Here's how the part is built. I have some questions about the finished solid (model axes, mm). A direction names the side the tool comes from. Coordinates: 2 decimals unless noted, no trailing zeros. Loops run counter-clockwise (first coordinate to the right, second up) from the corner with the lowest first, then second, coordinate; pieces in that order, holes last. Notation, with made-up numbers: (49.25, 85.5) -> (71.25, 85.5) arc R21 cw to (71.25, 101.5) -> close; hole circle Ø8 at (22.25, 38.5). An arc over 180 degrees is marked (long way). Use CSV: the item, a comma, the result in double quotes. Start each with the question number.
Autodesk Inventor part; units mm, degrees
ref_plane "YZ Plane" through (0, 0, 0) normal (1, 0, 0) x (0, 1, 0)
ref_plane "XZ Plane" through (0, 0, 0) normal (0, 1, 0) x (-1, 0, 0)
ref_plane "XY Plane" through (0, 0, 0) normal (0, 0, 1) x (1, 0, 0)
sketch "Sketch5" plane through (0, 0, 0) normal (0, 0, 1) x (1, 0, 0)
  line L0 (52.8, -15.6) -> (52.8, -10.6)
  line L1 (52.8, -10.6) -> (49.8, -10.6)
  line L2 (49.8, -10.6) -> (49.8, -12.55)
  line L3 (44, -12.55) -> (44, -3.05)
  line L4 (49.8, -3.05) -> (49.8, -5)
  line L5 (49.8, -5) -> (52.8, -5)
  line L6 (52.8, -5) -> (52.8, 0)
  line L7 (52.8, 0) -> (7.8, 0)
  line L8 (44, -3.05) -> (49.8, -3.05)
  line L9 (44, -12.55) -> (49.8, -12.55)
  line L10 (52.8, -15.6) -> (7.8, -15.6)
  arc A0 (7.8, 0) -> (7.8, -15.6) centre (7.8, -7.8) ccw
  point P0 (0, 0)
  dimension "d41" = 5.8
  dimension "d48" = 44
  dimension "d50" = 3
  dimension "d63" = 45
  dimension "d67" = 15.6
  dimension "d71" = 0
  dimension "d72" = 36.2
  dimension "d87" = 5.6
  dimension "d88" = 9.5
extrude "Extrusion2" add sketch "Sketch5" along normal blind 12
sketch "Sketch11" plane through (0, 0, 12) normal (0, 0, 1) x (1, 0, 0)
  line L0 (52.8, 0) -> (7.8, 0)
  line L1 (13.859, 0) -> (15.2481, -7.8785)
  line L2 (15.2481, -7.8785) -> (0.476, -10.4832)
  arc A0 (7.8, 0) -> (7.8, -15.6) centre (7.8, -7.8) ccw
  point P0 (0, 0)
  dimension "d95" = 100
  dimension "d96" = 8
  dimension "d97" = 15
extrude "Extrusion7" cut sketch "Sketch11" along normal blind 10 from surface at -12
sketch "Sketch14" plane through (0, 0, 12) normal (0, 0, 1) x (1, 0, 0)
  line L0 (2.8531, 4.8295) -> (7.1439, -19.5045)
  line L1 (7.1439, -19.5045) -> (-13.8708, -23.21)
  line L2 (-13.8708, -23.21) -> (-18.1616, 1.124)
  line L3 (-18.1616, 1.124) -> (2.8531, 4.8295)
  line L4 (13.859, 0) -> (15.2481, -7.8785)
  point P0 (0, 0)
  dimension "d111" = 10
extrude "Extrusion10" cut sketch "Sketch14" against normal through all
fillet "Fillet2" radius 15 1 edges at (6.4341, -15.4795, 6)
equation "\"l1\" = 8"
properties part number "Finray_test_8_Kerbe_10deg_V4"
1) Which directions (+Z, -Z, +X, -X, +Y, -Y) give clear straight access to the entire face, cutting with the end or side of a thin tool? Please do faces 4 (the face through (4.077, -2.113, 11.014)), 5 (the face through (44, -8, 6)), 6 (the face through (14.544, -3.884, 4.93)), 7 (the face through (51, -5, 6)), 8 (the face through (52.8, -3, 6)).
2) I want a section at A-A, the plane y = -4. Please give me the cut outline in (x, z).
3) For P1, Ø3, axis at x = 7, y = -3.5, coming from the -Z side; P2, Ø4, axis at y = -4.5, z = 8.5, coming from the -X side; P3, Ø2, axis at y = -4, z = 6.5, coming from the -X side, each with a flat end and sliding along its axis, tell me the tip position at first contact or that it passes through.
4) Please list where these lines run through material, in increasing order: L1, parallel to Y at x = 45, z = 3.5; L2, parallel to Y at x = 51.5, z = 2; L3, parallel to X at y = -4.5, z = 10.5. Write a range as [from, to].
5) I want a section at B-B, the plane z = 7.25. Please give me the cut outline in (x, y).
6) I want a section at C-C, the plane y = -2. Please give me the cut outline in (x, z), plus the area to 3 significant figures.
7) Thinking about a two-plate mould opening in X: for faces 1 (the face through (49.8, -12, 6)), 2 (the face through (51, -10.6, 6)), 3 (the face through (52.8, -13, 6)), which applies, pulls with the +X half, pulls with the -X half, needs draft (parallel to the pull), parting line crosses it, or undercut?
Return value:
1,face 4,"+Z, -Z, -X, -Y"
1,face 5,"+Z, -Z"
1,face 6,"-Z, -X"
1,face 7,"+Z, -Z, +X"
1,face 8,"+Z, -Z, +X, +Y, -Y"
2,outline,"(4.43, 10) -> (14.56, 10) -> (14.56, 0) -> (44, 0) -> (44, 12) -> (4.43, 12) -> close; (49.8, 0) -> (52.8, 0) -> (52.8, 12) -> (49.8, 12) -> close"
3,P1,"stops at z = 10"
3,P2,"stops at x = 4.26"
3,P3,"stops at x = 14.39"
4,L1,"y = [-15.6, -12.55], [-3.05, 0]"
4,L2,"y = [-15.6, -10.6], [-5, 0]"
4,L3,"x = [4.56, 44], [49.8, 52.8]"
5,outline,"(6.86, -9.36) arc R15 ccw to (19.04, -15.6) -> (52.8, -15.6) -> (52.8, -10.6) -> (49.8, -10.6) -> (49.8, -12.55) -> (44, -12.55) -> (44, -3.05) -> (49.8, -3.05) -> (49.8, -5) -> (52.8, -5) -> (52.8, 0) -> (13.86, 0) -> (15.25, -7.88) -> close"
6,outline,"(4.06, 10) -> (14.21, 10) -> (14.21, 0) -> (52.8, 0) -> (52.8, 12) -> (4.06, 12) -> close"
6,area,"483 mm²"
7,face 1,"undercut"
7,face 2,"needs draft"
7,face 3,"pulls with the +X half"
